Here's the drawing with two shaded views (mm, measured from the low corner). I have some questions. Round coordinates to 2 decimals unless told otherwise and drop trailing zeros. Order: outer loops, then holes, each group sorted by start corner. A loop starts at its lowest first (then second) coordinate and runs counter-clockwise, first axis right, second up. Notation, with made-up numbers: (39, -31) -> (70, -31) arc R26 cw to (70, -12) -> close; hole circle Ø5 at (83.5, 4.5). An arc over 180 degrees is marked (long way). Answer in a Markdown table with one row per item.
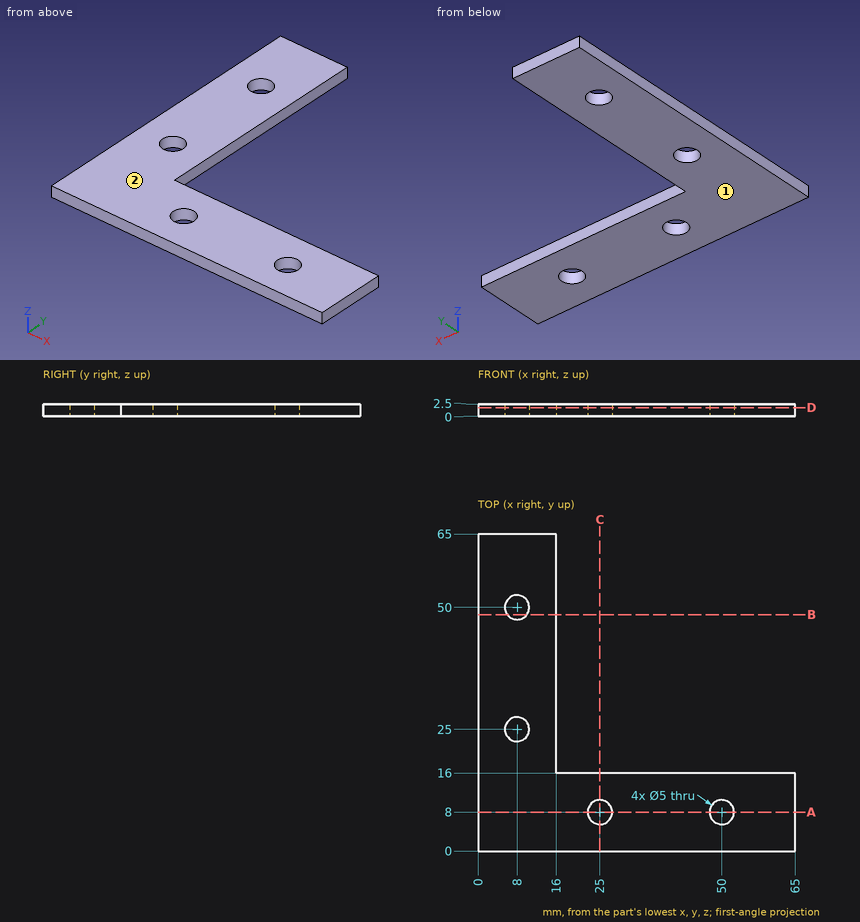
1. Suppose I cut it at B-B on y = 48.5. Write out the boundary of the cut face in (x, z), then the cut area to 3 significant figures.
Numbers:
| item | result |
|---|---|
| outline | (0, 0) -> (6, 0) -> (6, 2.5) -> (0, 2.5) -> close; (10, 0) -> (16, 0) -> (16, 2.5) -> (10, 2.5) -> close |
| area | 30.0 mm2 |
2. For pin 1 Ø4.5 at (x, y) = (8, 50) entering from +Z; pin 2 Ø1.2 at (y, z) = (30.5, 2) entering from +X; pin 3 Ø0.8 at (x, z) = (49, 1.5) entering from +Y, each with a flat end and sliding along its axis, tell me the tip position at first contact or that it passes through.
Numbers:
| item | result |
|---|---|
| pin 1 | passes through |
| pin 2 | stops at x = 16 |
| pin 3 | stops at y = 16 |
3. Suppose I cut it at A-A on y = 8. Write out the boundary of the cut face in (x, z).
Numbers:
| item | result |
|---|---|
| outline | (0, 0) -> (22.5, 0) -> (22.5, 2.5) -> (0, 2.5) -> close; (27.5, 0) -> (47.5, 0) -> (47.5, 2.5) -> (27.5, 2.5) -> close; (52.5, 0) -> (65, 0) -> (65, 2.5) -> (52.5, 2.5) -> close |
4. Suppose I cut it at D-D on z = 1.75. Write out the boundary of the cut face in (x, y).
Numbers:
| item | result |
|---|---|
| outline | (0, 0) -> (65, 0) -> (65, 16) -> (16, 16) -> (16, 65) -> (0, 65) -> close; hole circle Ø5 at (8, 25); hole circle Ø5 at (8, 50); hole circle Ø5 at (25, 8); hole circle Ø5 at (50, 8) |
5. Suppose I cut it at C-C on x = 25. Write out the boundary of the cut face in (y, z).
Numbers:
| item | result |
|---|---|
| outline | (0, 0) -> (5.5, 0) -> (5.5, 2.5) -> (0, 2.5) -> close; (10.5, 0) -> (16, 0) -> (16, 2.5) -> (10.5, 2.5) -> close |
6. We'd pull the mould along Z, two halves only. Please class the marked faces 1 and 2: released by +Z, released by -Z, zero draft, split by the parting line, or undercut.
Numbers:
| item | result |
|---|---|
| face 1 | released by -Z |
| face 2 | released by +Z |
7. Please list where these lines run through material, in increasing order: line 1 along Y through (x, z) = (8, 1.9); line 2 along Y through (x, z) = (50, 1.8); line 3 along X through (y, z) = (9.5, 0.5).
Numbers:
| item | result |
|---|---|
| line 1 | y = 0 to 22.5, 27.5 to 47.5, 52.5 to 65 |
| line 2 | y = 0 to 5.5, 10.5 to 16 |
| line 3 | x = 0 to 23, 27 to 48, 52 to 65 |
